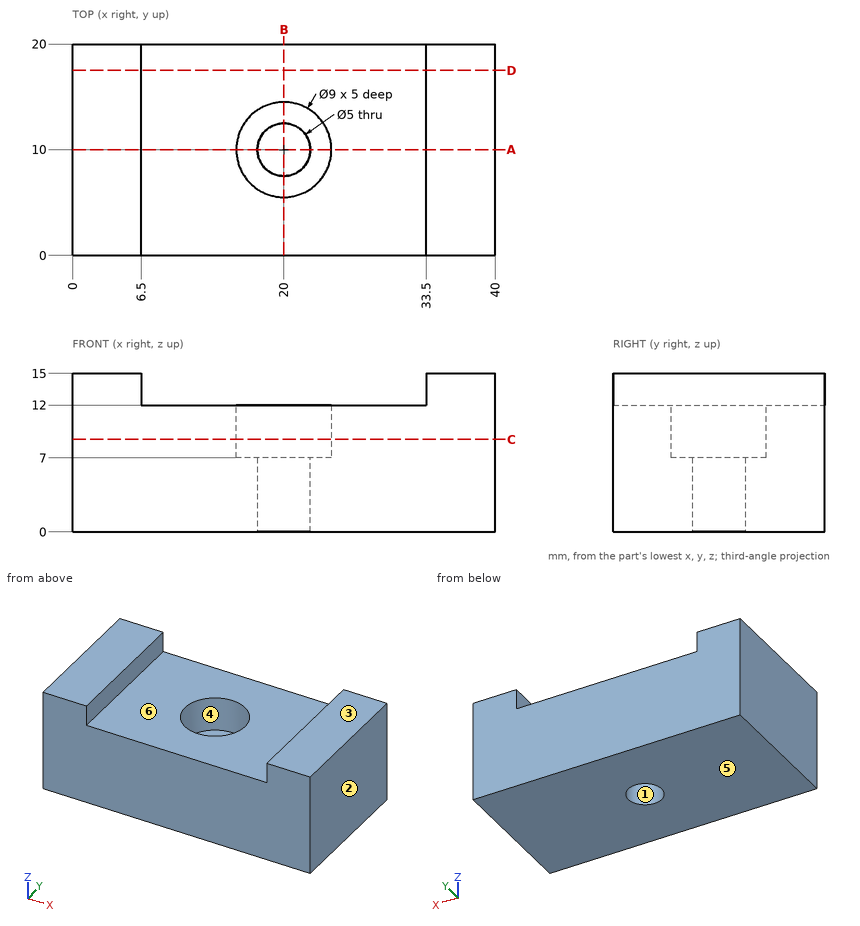
Could you check a few things on this drawing? It's one solid part, dimensions in mm from its lowest x, y, z. A direction names the side the tool comes from. Round coordinates to 2 decimals unless told otherwise and drop trailing zeros. Write each loop counter-clockwise with the first axis right and the second up, starting at its lowest first coordinate (ties: lowest second). Pieces come first, ordered by that corner, then holes.
Q1. If we section it at C-C on z = 8.75: Write out the boundary of the cut face in (x, y), plus the area to 3 significant figures.
Q2. If we section it at A-A on y = 10: Write out the boundary of the cut face in (x, z).
Q3. If we mould it in two halves opening along X, with no side actions, what happens to the marked faces 1, 2 and 3? For each: +X half, -X half, draft (parallel to the pull), parting line (faces both ways), or undercut.
Q4. Will these pins go through, and if not, where does the flat tip stop? P1, Ø1.5, axis at x = 18.5, y = 2.5, coming from the +Z side; P2, Ø4.5, axis at x = 21.5, y = 9.5, coming from the +Z side.
Q5. If we section it at D-D on y = 17.5: Write out the boundary of the cut face in (x, z).
Q6. Please list where these lines run through material, in increasing order: probe 1 along Y at (x, z) = (20, 5); probe 2 along X at (y, z) = (13.25, 14.25); probe 3 along X at (y, z) = (10, 4.5).
Q7. Which directions (+Z, -Z, +X, -X, +Y, -Y) give clear straight access to the entire face, cutting with the end or side of a thin tool? Please do the marked faces 4, 5 and 6.
Q8. If we section it at B-B on x = 20: Write out the boundary of the cut face in (y, z).
Answer below:
1. outline: (0, 0) - (40, 0) - (40, 20) - (0, 20) - close; hole circle Ø9 at (20, 10)
1. area: 736 mm2
2. outline: (0, 0) - (17.5, 0) - (17.5, 7) - (15.5, 7) - (15.5, 12) - (6.5, 12) - (6.5, 15) - (0, 15) - close; (22.5, 0) - (40, 0) - (40, 15) - (33.5, 15) - (33.5, 12) - (24.5, 12) - (24.5, 7) - (22.5, 7) - close
3. face 1: undercut
3. face 2: +X half
3. face 3: draft
4. P1: stops at z = 12
4. P2: stops at z = 7
5. outline: (0, 0) - (40, 0) - (40, 15) - (33.5, 15) - (33.5, 12) - (6.5, 12) - (6.5, 15) - (0, 15) - close
6. probe 1: y = 0 to 7.5, 12.5 to 20
6. probe 2: x = 0 to 6.5, 33.5 to 40
6. probe 3: x = 0 to 17.5, 22.5 to 40
7. face 4: +Z
7. face 5: -Z, +X, -X, +Y, -Y
7. face 6: +Z, +Y, -Y
8. outline: (0, 0) - (7.5, 0) - (7.5, 7) - (5.5, 7) - (5.5, 12) - (0, 12) - close; (12.5, 0) - (20, 0) - (20, 12) - (14.5, 12) - (14.5, 7) - (12.5, 7) - close
